```python
from build123d import *

# Parameters (mm, degrees)
SKETCH1_R           = 56
EXTRUDE1_DEPTH      = 69.5
SKETCH2_R           = 40
EXTRUDE2_DEPTH      = 25
EXTRUDE2_DEPTH_BACK = 3
SKETCH3_R           = 2.5
CUT_EXTRUDE1_DEPTH  = 10
SKETCH4_R           = 6.35
EXTRUDE3_DEPTH      = 12.7


with BuildPart() as part:
    # Sketch1 → Extrude1 (new body)
    with BuildSketch(Plane.XY):
        Circle(SKETCH1_R)
    extrude(amount=EXTRUDE1_DEPTH)

    # Sketch2 → Extrude2 (add, two sides)
    with BuildSketch(Plane(origin=(0, 0, 0), x_dir=(-1, 0, 0), z_dir=(0, 0, -1))) as extrude2_sk:
        with Locations((0, -36)):
            Circle(SKETCH2_R)
    extrude(amount=EXTRUDE2_DEPTH)
    extrude(extrude2_sk.sketch, amount=-EXTRUDE2_DEPTH_BACK)

    # Sketch3 → Cut-Extrude1 (cut)
    with BuildSketch(Plane(origin=(0, 0, 0), x_dir=(-1, 0, 0), z_dir=(0, 0, -1))):
        with Locations((-49, 0)):
            Circle(SKETCH3_R)
        with Locations((0, 49)):
            Circle(SKETCH3_R)
        with Locations((49, 0)):
            Circle(SKETCH3_R)
    extrude(amount=-CUT_EXTRUDE1_DEPTH, mode=Mode.SUBTRACT)

    # Sketch4 → Extrude3 (add)
    with BuildSketch(Plane(origin=(0, 0, -25), x_dir=(-1, 0, 0), z_dir=(0, 0, -1))):
        with Locations((0, -36)):
            Circle(SKETCH4_R)
    extrude(amount=EXTRUDE3_DEPTH)


solid = part.part
```
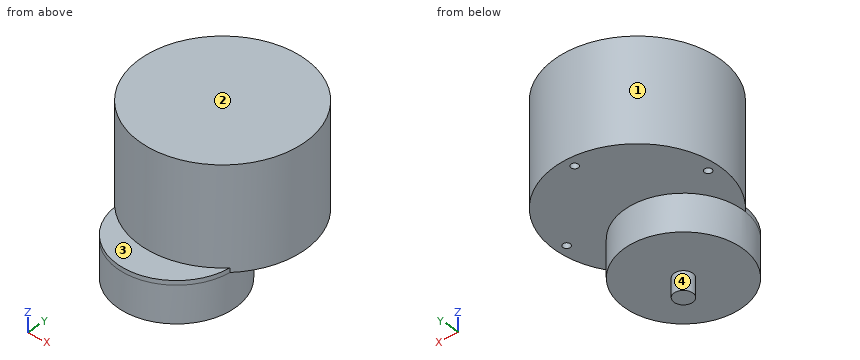
Geometry: final body of the model. Coordinates: model frame, mm. Face numbers are marked on the shaded views. A direction names the side the tool comes from. Round coordinates to 2 decimals unless told otherwise and drop trailing zeros. Write each loop counter-clockwise with the first axis right and the second up, starting at its lowest first coordinate (ties: lowest second). Pieces come first, ordered by that corner, then holes. Notation, with made-up numbers: (-12, 11) -> (19, 11) arc R13 cw to (19, 33) -> close; hole circle Ø9 at (-5.5, 85.25). An arc over 180 degrees is marked (long way). Use CSV: the item, a comma, the result in double quotes. Start each with the question number.
Q1. Section D-D (y = -36). Return loops of the section in (x, z), plus the area to 3 significant figures.
Q2. Section A-A (x = -15). Return loops of the section in (y, z), plus the area to 3 significant figures.
Q3. Line query: L1, parallel to Y at x = 0, z = 5.5; L2, parallel to Z at x = 31, y = 37; L3, parallel to Z at x = -22, y = -45. Output: solid intervals per line, ascending.
Q4. Section B-B (y = 0). Return loops of the section in (x, z), plus the area to 3 significant figures.
Q5. Reachability of the marked faces 1, 2, 3 and 4 from +Z, -Z, +X, -X, +Y, -Y: full face, straight path, thin tool, end or side. Return the list, or none.
Q6. Section C-C (z = 41). Return loops of the section in (x, y), plus the area to 3 significant figures.
Q7. First-contact query: pin 1 Ø3 at (y, z) = (-16.5, 34) entering from +X; pin 2 Ø12 at (x, z) = (-32.5, 36) entering from -Y; pin 3 Ø4 at (x, y) = (49, 0) entering from -Z. Flat tips, straight axial feed; report the tip coordinate or a pass-through.
Result sheet:
1,outline,"(-42.9, 0) -> (-40, 0) -> (-40, -25) -> (-6.35, -25) -> (-6.35, -37.7) -> (6.35, -37.7) -> (6.35, -25) -> (40, -25) -> (40, 0) -> (42.9, 0) -> (42.9, 69.5) -> (-42.9, 69.5) -> close"
1,area,"8,120 mm²"
2,outline,"(-73.08, -25) -> (1.08, -25) -> (1.08, 0) -> (53.95, 0) -> (53.95, 69.5) -> (-53.95, 69.5) -> (-53.95, 3) -> (-73.08, 3) -> close"
2,area,"9,410 mm²"
3,L1,"-56 to 46.5, 51.5 to 56"
3,L2,"0 to 69.5"
3,L3,"-25 to 69.5"
4,outline,"(-56, 0) -> (-51.5, 0) -> (-51.5, 10) -> (-46.5, 10) -> (-46.5, 0) -> (-17.44, 0) -> (-17.44, -25) -> (17.44, -25) -> (17.44, 0) -> (46.5, 0) -> (46.5, 10) -> (51.5, 10) -> (51.5, 0) -> (56, 0) -> (56, 69.5) -> (-56, 69.5) -> close"
4,area,"8,560 mm²"
5,face 1,"+Z"
5,face 2,"+Z, +X, -X, +Y, -Y"
5,face 3,"+Z, -Y"
5,face 4,"-Z"
6,outline,"circle Ø112 at (0, 0)"
6,area,"9,850 mm²"
7,pin 1,"x = 53.95"
7,pin 2,"y = -49.33"
7,pin 3,"z = 10"
